Input: part model. Units: mm. Frame: model coordinates. Give positions to 0.01 mm unless a question says otherwise; leave off trailing zeros. Loops run counter-clockwise (first coordinate to the right, second up) from the corner with the lowest first, then second, coordinate; pieces in that order, holes last. Notation, with made-up numbers: (39.25, 72) - (59.25, 72) arc R19 ccw to (59.25, 87) - close; hole circle Ø3 at (86.5, 22.25). An arc over 180 degrees is marked (long way). One line per question, with ' | ' between items. Start each with the question number.
from build123d import *

# Parameters (mm, degrees)
CAP_DISC_SKETCH_R                   = 20
CAP_DISC_DEPTH                      = 2.5
SHAFT_AND_SPACER_CLEARANCE_SKETCH_R = 11
SHAFT_AND_SPACER_CLEARANCE_DEPTH    = 2.7
M3_CAP_CLEARANCE_PATTERN_SKETCH_R   = 1.6
M3_CAP_CLEARANCE_PATTERN_DEPTH      = 2.7


with BuildPart() as part:
    # Cap disc sketch → Cap disc (new body)
    with BuildSketch(Plane(origin=(0, -240, 0), x_dir=(1, 0, 0), z_dir=(0, 1, 0))):
        with Locations(Location((-19.009182883, 53.244882879, 0), (0, 0, 270))):
            Circle(CAP_DISC_SKETCH_R)
    extrude(amount=CAP_DISC_DEPTH)

    # Shaft and spacer clearance sketch → Shaft and spacer clearance (cut)
    with BuildSketch(Plane(origin=(0, -240.1, 0), x_dir=(1, 0, 0), z_dir=(0, 1, 0))):
        with Locations(Location((-19.009182883, 53.244882879, 0), (0, 0, 90))):
            Circle(SHAFT_AND_SPACER_CLEARANCE_SKETCH_R)
    extrude(amount=SHAFT_AND_SPACER_CLEARANCE_DEPTH, mode=Mode.SUBTRACT)

    # M3 cap clearance pattern sketch → M3 cap clearance pattern (cut)
    with BuildSketch(Plane(origin=(0, -240.1, 0), x_dir=(1, 0, 0), z_dir=(0, 1, 0))):
        with Locations(Location((-6.493392856, 40.729092852, 0), (0, 0, 90))):
            Circle(M3_CAP_CLEARANCE_PATTERN_SKETCH_R)
        with Locations(Location((-31.52497291, 40.729092852, 0), (0, 0, 90))):
            Circle(M3_CAP_CLEARANCE_PATTERN_SKETCH_R)
        with Locations(Location((-31.52497291, 65.760672906, 0), (0, 0, 90))):
            Circle(M3_CAP_CLEARANCE_PATTERN_SKETCH_R)
        with Locations(Location((-6.493392856, 65.760672906, 0), (0, 0, 90))):
            Circle(M3_CAP_CLEARANCE_PATTERN_SKETCH_R)
    extrude(amount=M3_CAP_CLEARANCE_PATTERN_DEPTH, mode=Mode.SUBTRACT)


solid = part.part
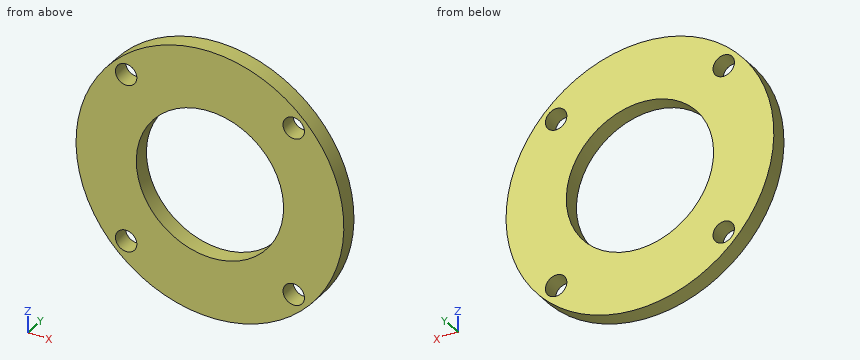
Q1. Section C-C, the plane z = -41.5. Output: boundary loops of the cut face in (x, y), plus the area to 3 significant figures.
Q2. Line query: L1, parallel to Z at x = -19, y = -238.35; L2, parallel to X at y = -239.1, z = -39.5; L3, parallel to X at y = -238.25, z = -41.5. Output: solid intervals per line, ascending. Write a range as from..to.
Q3. Section A-A, the plane z = -59. Output: boundary loops of the cut face in (x, y), plus the area to 3 significant figures.
Q4. First-contact query: pin 1 (1.9 mm diameter, centred on x = -6.49, z = -40.73, fed in from +Y); pin 2 (1.5 mm diameter, centred on y = -239, z = -56.5, fed in from -X). Flat tips, straight axial feed; report the tip coordinate or a pass-through.
Q5. Section B-B, the plane x = -18. Output: boundary loops of the cut face in (y, z).
Q6. Section D-D, the plane y = -238. Output: boundary loops of the cut face in (x, z).
Solved:
1) outline: (-35.2, -240) - (-32.93, -240) - (-32.93, -237.5) - (-35.2, -237.5) - close; (-30.12, -240) - (-7.9, -240) - (-7.9, -237.5) - (-30.12, -237.5) - close; (-5.09, -240) - (-2.82, -240) - (-2.82, -237.5) - (-5.09, -237.5) - close | area: 66.9 mm²
2) L1: z = -73.24..-64.24, -42.24..-33.24 | L2: x = -33.54..-32.55, -30.5..-7.52, -5.47..-4.48 | L3: x = -35.2..-32.93, -30.12..-7.9, -5.09..-2.82
3) outline: (-38.16, -240) - (-28.38, -240) - (-28.38, -237.5) - (-38.16, -237.5) - close; (-9.63, -240) - (0.14, -240) - (0.14, -237.5) - (-9.63, -237.5) - close | area: 48.9 mm²
4) pin 1: passes through | pin 2: stops at x = -38.85
5) outline: (-240, -73.22) - (-237.5, -73.22) - (-237.5, -64.2) - (-240, -64.2) - close; (-240, -42.29) - (-237.5, -42.29) - (-237.5, -33.27) - (-240, -33.27) - close
6) outline: circle Ø40 at (-19.01, -53.24); hole circle Ø3.2 at (-31.52, -65.76); hole circle Ø3.2 at (-31.52, -40.73); hole circle Ø22 at (-19.01, -53.24); hole circle Ø3.2 at (-6.49, -65.76); hole circle Ø3.2 at (-6.49, -40.73)
